from build123d import *

# Parameters (mm, degrees)
SKETCH1_W      = 360
SKETCH1_H      = 140
SKETCH1_R      = 15.5
EXTRUDE1_DEPTH = 12
SKETCH2_W      = 475
SKETCH2_H      = 12
EXTRUDE2_DEPTH = 183
SKETCH3_R      = 15.5
EXTRUDE3_DEPTH = 183
SKETCH4_W      = 12
SKETCH4_H      = 116
EXTRUDE4_DEPTH = 171
EXTRUDE5_DEPTH = 183


with BuildPart() as part:
    # Sketch1 → Extrude1 (new body)
    with BuildSketch(Plane.XY):
        with Locations((180, 70)):
            Rectangle(SKETCH1_W, SKETCH1_H)
        with Locations((80, 95)):
            Circle(SKETCH1_R, mode=Mode.SUBTRACT)
        with Locations((180, 95)):
            Circle(SKETCH1_R, mode=Mode.SUBTRACT)
        with Locations((280, 95)):
            Circle(SKETCH1_R, mode=Mode.SUBTRACT)
    extrude(amount=EXTRUDE1_DEPTH)

    # Sketch2 → Extrude2 (add)
    with BuildSketch(Plane.XY.offset(12)):
        with Locations((180, 6)):
            Rectangle(SKETCH2_W, SKETCH2_H)
    extrude(amount=EXTRUDE2_DEPTH)

    # Sketch3 → Extrude3 (cut)
    with BuildSketch(Plane(origin=(0, 12, 0), x_dir=(1, 0, 0), z_dir=(0, 1, 0))):
        Polygon((360, -12), (417.5, -62), (417.5, -12), align=None)
        Polygon((417.5, -165), (387.5, -195), (417.5, -195), align=None)
        Polygon((-57.5, -165), (-57.5, -195), (-27.5, -195), align=None)
        Polygon((-57.5, -12), (-57.5, -62), (0, -12), align=None)
        with Locations(Location((58.413652083, -91.738221798, 0), (0, 0, 270))):
            Circle(SKETCH3_R)
        with Locations(Location((-11.732317869, -148.125657451, 0), (0, 0, 270))):
            Circle(SKETCH3_R)
        with Locations(Location((301.586347917, -91.738221798, 0), (0, 0, 270))):
            Circle(SKETCH3_R)
        with Locations(Location((371.732317869, -148.125657451, 0), (0, 0, 270))):
            Circle(SKETCH3_R)
    extrude(amount=-EXTRUDE3_DEPTH, mode=Mode.SUBTRACT)

    # Sketch4 → Extrude4 (add)
    with BuildSketch(Plane.XY.offset(12)):
        with Locations((130, 70)):
            Rectangle(SKETCH4_W, SKETCH4_H)
        with Locations((230, 70)):
            Rectangle(SKETCH4_W, SKETCH4_H)
    extrude(amount=EXTRUDE4_DEPTH)

    # Sketch5 → Extrude5 (cut)
    with BuildSketch(Plane.ZY.offset(-124)):
        Polygon((183, 128), (183, 24), (24, 128), align=None)
    extrude(amount=-EXTRUDE5_DEPTH, mode=Mode.SUBTRACT)


solid = part.part
Can you work these out from the model? Positions are in its coordinate system, mm. A direction names the side the tool comes from. Coordinates: 2 decimals unless noted, no trailing zeros. Loops run counter-clockwise (first coordinate to the right, second up) from the corner with the lowest first, then second, coordinate; pieces in that order, holes last. Notation, with made-up numbers: M 25.5,3 L 52.5,3 A26 cw 52.5,22 Z; hole C 74.25,9 d9. An arc over 180 degrees is marked long. Answer as CSV lines item,"result". Start each with the question number.
1. For pin 1 Ø13 at (y, z) = (81, 7.5) entering from +X; pin 2 Ø10 at (x, y) = (210, 99) entering from +Z; pin 3 Ø9.5 at (x, z) = (127.5, 18.5) entering from +Y; pin 4 Ø25 at (x, y) = (80, 95) entering from -Z, each with a flat end and sliding along its axis, tell me the tip position at first contact or that it passes through.
2. Suppose I cut it at D-D, the plane x = 153. List the corners of the cut face in (y, z) for me, plus the area to 3 significant figures.
3. Thinking about a two-plate mould opening in Z: for faces 6 (the face through (136, 56, 77)), 7 (the face through (295.65, 6.084, 106.056)), 8 (the face through (-29.15, 6.08, 37.35)), 9 (the face through (177, 6, 195)), which applies, +Z half, -Z half, draft (parallel to the pull), parting line (faces both ways), or undercut?
4. Suppose I cut it at B-B, the plane z = 158. List the corners of the cut face in (x, y) for me, plus the area to 3 significant figures.
5. Suppose I cut it at A-A, the plane x = 280. List the corners of the cut face in (y, z) for me.
6. If I drill on probe 1 along Y at (x, z) = (80, 4); probe 2 along X at (y, z) = (80, 32); probe 3 along Y at (x, z) = (89, 84), over which ranges is the centre line in solid material (lowest first)? Write a range as [from, to].
7. Suppose I cut it at C-C, the plane y = 117. List the corners of the cut face in (x, z) for me.
8. For faces 1 (the face through (124, 56, 77)), 2 (the face through (224, 56, 77)), 3 (the face through (164.515, 95.682, 5.916)), 4 (the face through (177, 140, 6)), 5 (the face through (130, 18, 183)), which set-ups out of +Z, -Z, +X, -X, +Y, -Y let a thin tool reach every point of the face, with its end or its side?
Output:
1,pin 1,"stops at x = 360"
1,pin 2,"stops at z = 12"
1,pin 3,"stops at y = 128"
1,pin 4,"passes through"
2,outline,"M 0,0 L 140,0 L 140,12 L 12,12 L 12,195 L 0,195 Z"
2,area,"3,880 mm^2"
3,face 6,"draft"
3,face 7,"undercut"
3,face 8,"-Z half"
3,face 9,"+Z half"
4,outline,"M -57.5,0 L -23.68,0 L -23.68,12 L -57.5,12 Z; M 0.22,0 L 359.78,0 L 359.78,12 L 236,12 L 236,40.35 L 224,40.35 L 224,12 L 136,12 L 136,40.35 L 124,40.35 L 124,12 L 0.22,12 Z; M 383.68,0 L 417.5,0 L 417.5,12 L 383.68,12 Z"
4,area,"5,810 mm^2"
5,outline,"M 0,0 L 79.5,0 L 79.5,12 L 12,12 L 12,195 L 0,195 Z; M 110.5,0 L 140,0 L 140,12 L 110.5,12 Z"
6,probe 1,"y = [0, 79.5], [110.5, 140]"
6,probe 2,"x = [124, 136], [224, 236]"
6,probe 3,"y = [0, 12]"
7,outline,"M 0,0 L 360,0 L 360,12 L 236,12 L 236,40.82 L 224,40.82 L 224,12 L 136,12 L 136,40.82 L 124,40.82 L 124,12 L 0,12 Z"
8,face 1,"+Z, -X, +Y"
8,face 2,"+Z, +Y"
8,face 3,"+Z, -Z"
8,face 4,"+Z, -Z, +X, -X, +Y"
8,face 5,"+Z, +X, -X, +Y"
